from build123d import *

# Parameters (mm, degrees)
F0_W          = 58
F0_H          = 6
F0_R          = 1.5
F1_DEPTH      = 1
F1_DEPTH_BACK = 1


with BuildPart() as f1:
    # F0 (on Right) → F1 (new body, two sides)
    with BuildSketch(Plane.YZ) as f1_sk:
        Rectangle(F0_W, F0_H)
        with Locations((-26, 0)):
            Circle(F0_R, mode=Mode.SUBTRACT)
        with Locations((26, 0)):
            Circle(F0_R, mode=Mode.SUBTRACT)
    extrude(amount=F1_DEPTH)
    extrude(f1_sk.sketch, amount=-F1_DEPTH_BACK)


solid = f1.part
Input: part model. Units: mm. Frame: model coordinates. Give positions to 0.01 mm unless a question says otherwise; leave off trailing zeros. Order: outer loops, then holes, each group sorted by start corner. A loop starts at its lowest first (then second) coordinate and runs counter-clockwise, first axis right, second up. Notation, with made-up numbers: (68.25, 82.25) - (106.25, 82.25) arc R23 cw to (106.25, 92.25) - close; hole circle Ø11 at (40, 82). An arc over 180 degrees is marked (long way). Answer as a JSON object with one key per item and string values. Group by question number.
Q1. First-contact query: pin 1 Ø2.5 at (y, z) = (26, 0) entering from +X. Flat tip, straight axial feed; report the tip coordinate or a pass-through.
Q2. Cut plane B-B, the plane y = -26. Output: boundary loops of the cut face in (x, z).
Q3. Cut plane A-A, the plane z = 0. Output: boundary loops of the cut face in (x, y).
Q4. Line query: probe 1 along Z at (x, y) = (0.5, 26); probe 2 along Y at (x, z) = (0.6, -0.55); probe 3 along Z at (x, y) = (0, -25). Output: solid intervals per line, ascending.
Q5. Cut plane C-C, the plane x = 0.6. Output: boundary loops of the cut face in (y, z).
Q6. Mould query, pull axis Z, two halves, no side actions, for faces 1 (the face through (0, 0, 3)), 2 (the face through (-0.01, -27.5, 0.07)), 3 (the face through (-1, 0, 0)). Classes: pulls with the +Z half, pulls with the -Z half, needs draft (parallel to the pull), parting line crosses it, or undercut.
Results:
{
 "1": {"pin 1": "through"},
 "2": {"outline": "(-1, -3) - (1, -3) - (1, -1.5) - (-1, -1.5) - close; (-1, 1.5) - (1, 1.5) - (1, 3) - (-1, 3) - close"},
 "3": {"outline": "(-1, -29) - (1, -29) - (1, -27.5) - (-1, -27.5) - close; (-1, -24.5) - (1, -24.5) - (1, 24.5) - (-1, 24.5) - close; (-1, 27.5) - (1, 27.5) - (1, 29) - (-1, 29) - close"},
 "4": {"probe 1": "-3 to -1.5, 1.5 to 3", "probe 2": "-29 to -27.4, -24.6 to 24.6, 27.4 to 29", "probe 3": "-3 to -1.12, 1.12 to 3"},
 "5": {"outline": "(-29, -3) - (29, -3) - (29, 3) - (-29, 3) - close; hole circle Ø3 at (-26, 0); hole circle Ø3 at (26, 0)"},
 "6": {"face 1": "pulls with the +Z half", "face 2": "undercut", "face 3": "needs draft"}
}
